For this review, take the finished solid that the model builds, in its own axes (mm). Coordinates: 2 decimals unless noted, no trailing zeros. Write each loop counter-clockwise with the first axis right and the second up, starting at its lowest first coordinate (ties: lowest second). Pieces come first, ordered by that corner, then holes.
1) We need section A-A on x = -20. Write out the cut boundary in (y, z).
2) To check wall thickness, follow line 1 along X through (y, z) = (91, 1.4); line 2 along X through (y, z) = (-76, 0.95); line 3 along Y through (x, z) = (-38.5, 0.6). State the ranges of each line that lie inside material, in increasing order.
3) Mouldability with a two-part tool opening along Y and no side actions: class faces 1 (the face through (-51.28, -91.04, 1.52)), 2 (the face through (37.243, 89.245, 1.479)), 3 (the face through (-51.97, -77.48, 1.48)), 4 (the face through (-1, 6, 3)) as pulls with the +Y half, pulls with the -Y half, needs draft (parallel to the pull), parting line crosses it, or undercut.
4) Insertion check: P1, Ø0.9, axis at x = -21, z = 1.5, coming from the +Y side; P2, Ø0.9, axis at y = 104, z = 1, coming from the +X side; P3, Ø1.8, axis at x = 34.9, y = -86.21, coming from the -Z side; P4, Ø1.5, axis at y = 105.5, z = 1.5, coming from the -X side. Each pin has a flat end and moves straight along its axis. Give the tip position at first contact, or say it passes through.
5) We need section B-B on z = 2.3. Give the number of separate pieces and of enclosed holes in the cut face, then the cut area to 3 significant figures.
Autodesk Inventor part; units mm, degrees
ref_plane "YZ Plane" through (0, 0, 0) normal (1, 0, 0) x (0, 1, 0)
ref_plane "XZ Plane" through (0, 0, 0) normal (0, 1, 0) x (-1, 0, 0)
ref_plane "XY Plane" through (0, 0, 0) normal (0, 0, 1) x (1, 0, 0)
sketch "スケッチ1" plane through (0, 0, 0) normal (0, 0, 1) x (1, 0, 0)
  line L0 (-60, 100) -> (60, 100)
  line L1 (60, 100) -> (60, -100)
  line L2 (60, -100) -> (-60, -100)
  line L3 (-60, -100) -> (-60, 100)
  line L4 (60, 117.6777) -> (77.6777, 100)
  line L5 (77.6777, 100) -> (60, 82.3223)
  line L6 (60, 82.3223) -> (42.3223, 100)
  line L7 (42.3223, 100) -> (60, 117.6777)
  line L8 (60, -82.3223) -> (77.6777, -100)
  line L9 (77.6777, -100) -> (60, -117.6777)
  line L10 (60, -117.6777) -> (42.3223, -100)
  line L11 (42.3223, -100) -> (60, -82.3223)
  line L12 (-60, -82.3223) -> (-42.3223, -100)
  line L13 (-42.3223, -100) -> (-60, -117.6777)
  line L14 (-60, -117.6777) -> (-77.6777, -100)
  line L15 (-77.6777, -100) -> (-60, -82.3223)
  line L16 (-60, 117.6777) -> (-42.3223, 100)
  line L17 (-42.3223, 100) -> (-60, 82.3223)
  line L18 (-60, 82.3223) -> (-77.6777, 100)
  line L19 (-77.6777, 100) -> (-60, 117.6777)
  point P0 (0, 0)
  dimension "d0" = 200
  dimension "d1" = 100
  dimension "d2" = 120
  dimension "d3" = 60
  dimension "d4" = 12.5
  dimension "d5" = 12.5
  dimension "d6" = 12.5
  dimension "d7" = 12.5
extrude "押し出し1" add sketch "スケッチ1" along normal blind 3
sketch "スケッチ2" plane through (0, 0, 3) normal (0, 0, 1) x (1, 0, 0)
  line L0 (77.6777, 100) -> (60, 82.3223)
  line L1 (60, 117.6777) -> (77.6777, 100)
  line L2 (42.3223, 100) -> (60, 117.6777)
  line L3 (-60, 117.6777) -> (-42.3223, 100)
  line L4 (-77.6777, 100) -> (-60, 117.6777)
  line L5 (-60, 82.3223) -> (-77.6777, 100)
  line L6 (-77.6777, -100) -> (-60, -82.3223)
  line L7 (-60, -117.6777) -> (-77.6777, -100)
  line L8 (-42.3223, -100) -> (-60, -117.6777)
  line L9 (60, -117.6777) -> (42.3223, -100)
  line L10 (77.6777, -100) -> (60, -117.6777)
  line L11 (60, -82.3223) -> (77.6777, -100)
  circle A0 centre (-46.2114, -74.8977) radius 1.5
  circle A1 centre (-34.8977, -86.2114) radius 1.5
  circle A2 centre (34.8977, -86.2114) radius 1.5
  circle A3 centre (46.2114, -74.8977) radius 1.5
  circle A4 centre (46.2114, 74.8977) radius 1.5
  circle A5 centre (34.8977, 86.2114) radius 1.5
  circle A6 centre (-34.8977, 86.2114) radius 1.5
  circle A7 centre (-46.2114, 74.8977) radius 1.5
  point P0 (0, 0)
  dimension "d10" = 3
  dimension "d12" = 40
  dimension "d13" = 40
  dimension "d14" = 4.5
  dimension "d15" = 4.5
  dimension "d16" = 40
  dimension "d17" = 40
  dimension "d18" = 40
  dimension "d19" = 40
  dimension "d20" = 40
  dimension "d21" = 40
  dimension "d22" = 4.5
  dimension "d23" = 4.5
  dimension "d24" = 4.5
  dimension "d25" = 4.5
  dimension "d26" = 4.5
  dimension "d27" = 4.5
hole "穴1" at (34.8977, -86.2114, 3) at (46.2114, -74.8977, 3) at (-34.8977, -86.2114, 3) at (-46.2114, -74.8977, 3) at (34.8977, 86.2114, 3) at (46.2114, 74.8977, 3) at (-46.2114, 74.8977, 3) at (-34.8977, 86.2114, 3) direction (0, 0, -1) diameter 3 end through all
sketch "スケッチ3" plane through (0, 0, 3) normal (0, 0, 1) x (1, 0, 0)
  line L0 (77.6777, 100) -> (60, 82.3223)
  line L1 (60, 117.6777) -> (77.6777, 100)
  line L2 (42.3223, 100) -> (60, 117.6777)
  line L3 (-60, 117.6777) -> (-42.3223, 100)
  line L4 (-77.6777, 100) -> (-60, 117.6777)
  line L5 (-60, 82.3223) -> (-77.6777, 100)
  line L6 (-77.6777, -100) -> (-60, -82.3223)
  line L7 (-60, -117.6777) -> (-77.6777, -100)
  line L8 (-42.3223, -100) -> (-60, -117.6777)
  line L9 (60, -117.6777) -> (42.3223, -100)
  line L10 (77.6777, -100) -> (60, -117.6777)
  line L11 (60, -82.3223) -> (77.6777, -100)
  circle A0 centre (-39.1403, 90.4541) radius 2.25
  circle A1 centre (-50.4541, 79.1403) radius 2.25
  circle A2 centre (-50.4541, -79.1403) radius 2.25
  circle A3 centre (-39.1403, -90.4541) radius 2.25
  circle A4 centre (39.1403, -90.4541) radius 2.25
  circle A5 centre (50.4541, -79.1403) radius 2.25
  circle A6 centre (50.4541, 79.1403) radius 2.25
  circle A7 centre (39.1403, 90.4541) radius 2.25
  point P0 (0, 0)
  dimension "d35" = 4.5
  dimension "d37" = 4.5
  dimension "d38" = 4.5
  dimension "d39" = 34
  dimension "d40" = 34
  dimension "d41" = 4.5
  dimension "d42" = 4.5
  dimension "d43" = 34
  dimension "d44" = 34
  dimension "d45" = 34
  dimension "d46" = 4.5
  dimension "d47" = 4.5
  dimension "d48" = 34
  dimension "d49" = 34
  dimension "d50" = 34
  dimension "d51" = 4.5
  dimension "d52" = 4.5
hole "穴2" at (-50.4541, -79.1403, 3) at (-39.1403, -90.4541, 3) at (39.1403, 90.4541, 3) at (50.4541, 79.1403, 3) at (-50.4541, 79.1403, 3) at (-39.1403, 90.4541, 3) at (39.1403, -90.4541, 3) at (50.4541, -79.1403, 3) direction (0, 0, -1) diameter 4.5 end through all
sketch "スケッチ4" plane through (0, 0, 3) normal (0, 0, 1) x (1, 0, 0)
  line L0 (77.6777, 100) -> (60, 82.3223)
  line L1 (60, 117.6777) -> (77.6777, 100)
  line L2 (42.3223, 100) -> (60, 117.6777)
  line L3 (-60, 117.6777) -> (-42.3223, 100)
  line L4 (-77.6777, 100) -> (-60, 117.6777)
  line L5 (-60, 82.3223) -> (-77.6777, 100)
  line L6 (-77.6777, -100) -> (-60, -82.3223)
  line L7 (-60, -117.6777) -> (-77.6777, -100)
  line L8 (-42.3223, -100) -> (-60, -117.6777)
  line L9 (60, -117.6777) -> (42.3223, -100)
  line L10 (77.6777, -100) -> (60, -117.6777)
  line L11 (60, -82.3223) -> (77.6777, -100)
  line L12 (-60, -82.3223) -> (-42.3223, -100)
  line L13 (42.3223, -100) -> (60, -82.3223)
  line L14 (42.3223, 100) -> (60, 82.3223)
  line L15 (-60, 82.3223) -> (-42.3223, 100)
  point P0 (0, 0)
  dimension "d60" = 25
  dimension "d61" = 25
  dimension "d62" = 25
  dimension "d63" = 25
extrude "押し出し2" cut sketch "スケッチ4" against normal blind 3
sketch "スケッチ6" plane through (-42.3223, 100, 0) normal (0, 1, 0) x (1, 0, 0)
  line L0 (84.6447, 0) -> (0, 0)
  line L1 (0, -3) -> (84.6447, -3)
  line L2 (29.8223, 0) -> (54.8223, 0)
  line L3 (54.8223, 0) -> (54.8223, -3)
  line L4 (54.8223, -3) -> (29.8223, -3)
  line L5 (29.8223, -3) -> (29.8223, 0)
  point P0 (42.3223, 0)
  dimension "d66" = 25
  dimension "d68" = 12.5
extrude "押し出し3" add sketch "スケッチ6" along normal blind 10
sketch "スケッチ7" plane through (0, 0, 3) normal (0, 0, 1) x (1, 0, 0)
  line L0 (-12.5, 110) -> (12.5, 110)
  line L1 (-12.5, 100) -> (-12.5, 110)
  circle A0 centre (-8, 98) radius 1.5
  circle A1 centre (8, 98) radius 1.5
  point P0 (0, 0)
  dimension "d71" = 16
  dimension "d72" = 12
  dimension "d73" = 12
  dimension "d74" = 3
  dimension "d75" = 4.5
hole "穴3" at (-8, 98, 3) at (8, 98, 3) direction (0, 0, -1) diameter 3 end through all
equation "\"d33\" = d26"
equation "\"d58\" = d46"
properties material "アルミニウム 6061"
Result:
1. outline: (-100, 0) - (100, 0) - (100, 3) - (-100, 3) - close
2. line 1: x = -51.32 to -41.32, -36.96 to 36.96, 41.32 to 51.32
2. line 2: x = -60 to -47.23, -45.19 to 45.19, 47.23 to 60
2. line 3: y = -100 to -92.61, -88.3 to 88.3, 92.61 to 100
3. face 1: pulls with the -Y half
3. face 2: undercut
3. face 3: undercut
3. face 4: needs draft
4. P1: stops at y = 100
4. P2: stops at x = 12.5
4. P3: passes through
4. P4: stops at x = -12.5
5. separate pieces: 1
5. enclosed holes: 18
5. area: 23,400 mm2
